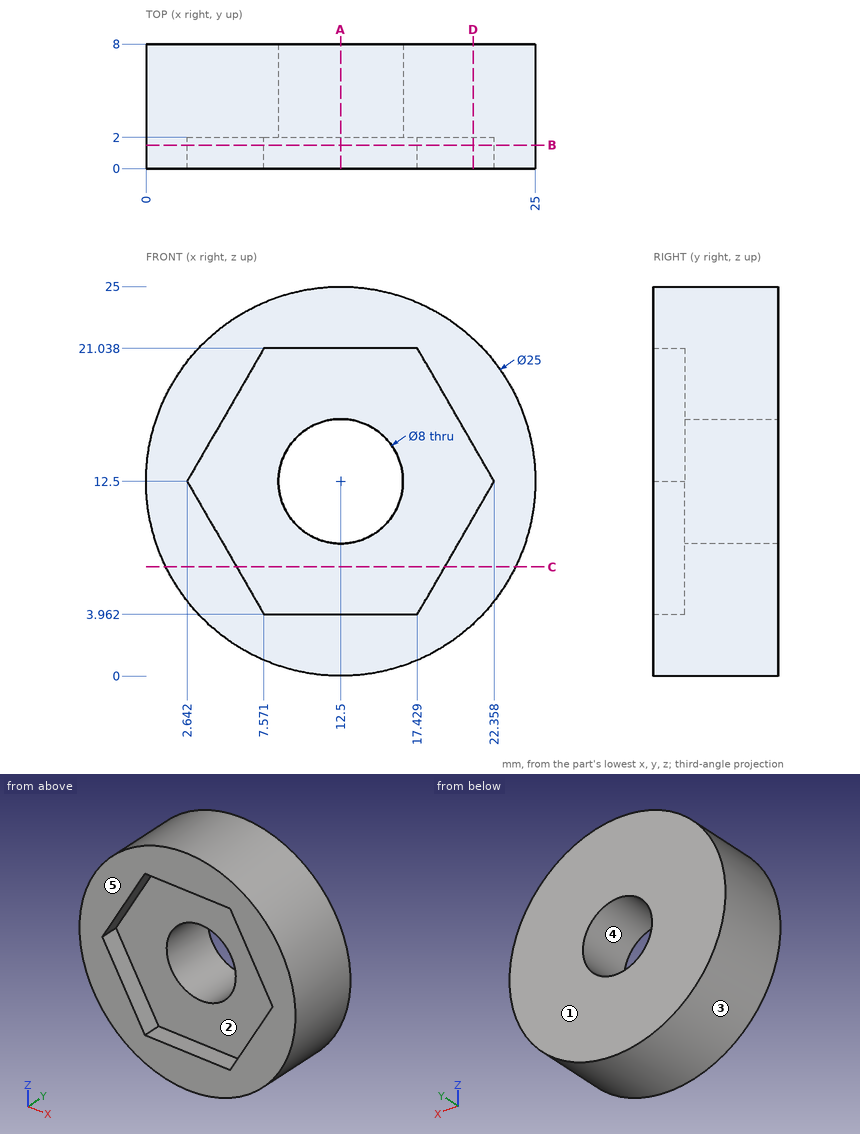
Part print with two shaded views. Sizes in mm from the minimum x, y, z corner. A direction names the side the tool comes from. Give positions to 0.01 mm unless a question says otherwise; leave off trailing zeros. Order: outer loops, then holes, each group sorted by start corner. A loop starts at its lowest first (then second) coordinate and runs counter-clockwise, first axis right, second up. Notation, with made-up numbers: M 38,57.5 L 80,57.5 A12 cw 80,73.5 Z; hole C 55.25,-14.5 d11. An arc over 180 degrees is marked long. Use one line per item in the form item = value.
1) Drop flat-ended pins along their axis: pin 1 (5 mm diameter, centred on x = 12.5, z = 12.5, fed in from +Y); pin 2 (2 mm diameter, centred on x = 20, y = 2.5, fed in from +Z); pin 3 (1.5 mm diameter, centred on x = 11.5, y = 6.5, fed in from +Z); pin 4 (5 mm diameter, centred on x = 13.5, z = 10.5, fed in from -Y). Give the stop position or say it passes through.
Calculated:
pin_1 = through
pin_2 = 23.18
pin_3 = 25
pin_4 = 2
2) Two-plate mould, pull along Z, no slides. Class the marked faces 3, 4 and 5: released by +Z, released by -Z, zero draft, split by the parting line, or undercut.
Calculated:
face_3 = split by the parting line
face_4 = undercut
face_5 = zero draft
3) Saw through at D-D (x = 21). Give the cut face in (y, z) (1 decimal), plus the area to 3 significant figures.
Calculated:
outline = M 0,3.3 L 8,3.3 L 8,21.7 L 0,21.7 L 0,14.9 L 2,14.9 L 2,10.1 L 0,10.1 Z
area = 137 mm2
4) Saw through at C-C (z = 7). Give the cut face in (x, y) (1 decimal), plus the area to 3 significant figures.
Calculated:
outline = M 1.3,0 L 5.8,0 L 5.8,2 L 19.2,2 L 19.2,0 L 23.7,0 L 23.7,8 L 1.3,8 Z
area = 153 mm2
5) Saw through at B-B (y = 1.5). Give the cut face in (x, z).
Calculated:
outline = C 12.5,12.5 d25; hole M 2.64,12.5 L 7.57,3.96 L 17.43,3.96 L 22.36,12.5 L 17.43,21.04 L 7.57,21.04 Z
6) Saw through at A-A (x = 12.5). Give the cut face in (y, z).
Calculated:
outline = M 0,0 L 8,0 L 8,8.5 L 2,8.5 L 2,3.96 L 0,3.96 Z; M 0,21.04 L 2,21.04 L 2,16.5 L 8,16.5 L 8,25 L 0,25 Z
7) Tool access for the marked faces 1 and 2: list every direction of +Z, -Z, +X, -X, +Y, -Y with a clear straight run to the whole face (end or side of a thin tool).
Calculated:
face_1 = +Z, -Z, +X, -X, +Y
face_2 = -Y
8) Probe probe 1 along X at (y, z) = (5.75, 12.5); probe 2 along Z at (x, y) = (12.25, 5.5); probe 3 along X at (y, z) = (4.25, 10.25) (1 decimal). List the from-to ranges inside material, lowest first.
Calculated:
probe_1 = 0 to 8.5, 16.5 to 25
probe_2 = 0 to 8.51, 16.49 to 25
probe_3 = 0.2 to 9.2, 15.8 to 24.8
